Here's how the part is built. I have some questions about the finished solid (model axes, mm). A direction names the side the tool comes from. Give positions to 0.01 mm unless a question says otherwise; leave off trailing zeros. Loops run counter-clockwise (first coordinate to the right, second up) from the corner with the lowest first, then second, coordinate; pieces in that order, holes last. Notation, with made-up numbers: (67, 78.25) - (81, 78.25) arc R21 ccw to (81, 114.25) - close; hole circle Ø7 at (-9, 68.25). An arc over 180 degrees is marked (long way). Put each result on its own line as item: value. Start each with the question number.
Autodesk Inventor part; units mm, degrees
ref_plane "YZ Plane" through (0, 0, 0) normal (1, 0, 0) x (0, 1, 0)
ref_plane "XZ Plane" through (0, 0, 0) normal (0, 1, 0) x (-1, 0, 0)
ref_plane "XY Plane" through (0, 0, 0) normal (0, 0, 1) x (1, 0, 0)
sketch "スケッチ1" plane through (0, 0, 0) normal (0, 0, 1) x (1, 0, 0)
  line L0 (0, 0) -> (80, 0)
  line L1 (80, 0) -> (80, 45)
  line L2 (80, 45) -> (0, 45)
  line L3 (0, 45) -> (0, 0)
  dimension "d0" = 80
  dimension "d1" = 45
extrude "押し出し1" add sketch "スケッチ1" along normal blind 3
sketch "スケッチ2" plane through (0, 0, 3) normal (0, 0, 1) x (1, 0, 0)
  line L0 (0, 45) -> (0, 0)
  line L1 (0, 0) -> (80, 0)
  line L2 (80, 45) -> (0, 45)
  line L3 (40, 45) -> (40, 0) construction
  point P0 (7.5, 35)
  point P1 (7.5, 25)
  point P2 (30, 7.5)
  point P3 (72.5, 35)
  point P4 (72.5, 25)
  point P5 (50, 7.5)
  point P6 (40, 7.5)
  dimension "d4" = 7.5
  dimension "d5" = 35
  dimension "d6" = 10
  dimension "d7" = 7.5
  dimension "d8" = 7.5
  dimension "d9" = 30
hole "穴1" at (7.5, 35, 3) at (7.5, 25, 3) at (30, 7.5, 3) at (72.5, 35, 3) at (72.5, 25, 3) at (50, 7.5, 3) at (40, 7.5, 3) direction (0, 0, -1) diameter 3.2 end through all
sketch "スケッチ3" plane through (0, 0, 3) normal (0, 0, 1) x (1, 0, 0)
  line L0 (80, 45) -> (0, 45)
  line L1 (15, 45) -> (65, 45)
  line L2 (65, 45) -> (65, 15)
  line L3 (65, 15) -> (15, 15)
  line L4 (15, 15) -> (15, 45)
  line L5 (0, 45) -> (0, 0)
  line L6 (0, 0) -> (80, 0)
  dimension "d17" = 50
  dimension "d18" = 30
  dimension "d19" = 15
  dimension "d20" = 15
extrude "押し出し2" cut sketch "スケッチ3" against normal blind 3
fillet "フィレット1" radius 2 8 edges at (15, 45, 1.5) (65, 15, 1.5) (65, 45, 1.5) (80, 45, 1.5) (0, 45, 1.5) (0, 0, 1.5) (80, 0, 1.5) (15, 15, 1.5)
properties part number "射出_固定1" material "アルミニウム 6061"
1) Which directions (+Z, -Z, +X, -X, +Y, -Y) give clear straight access to the entire face, cutting with the end or side of a thin tool? Please do faces 4 (the flat face through (65, 30, 2)), 5 (the cylindrical face through (70.914, 25.208, 1.479)).
2) I'm going to push a flat-ended pin straight in: P1, Ø3, axis at x = 40, y = 7.5, coming from the +Z side. Where does the tip first touch, or does it pass through?
3) Suppose I cut it at B-B on y = 7.5. Please give me the cut outline in (x, z).
4) Suppose I cut it at D-D on z = 2.2. Please give me the cut outline in (x, y).
5) Suppose I cut it at A-A on y = 30. Please give me the cut outline in (x, z).
6) I need wall thicknesses on line 1 (X direction, y = 7.5, z = 2.1); line 2 (Y direction, x = 7.5, z = 1.5); line 3 (Y direction, x = 40, z = 1.3). Which ranges of each line are inside material? Lowest first, please.
7) Suppose I cut it at C-C on x = 30. Please give me the cut outline in (y, z).
8) Thinking about a two-plate mould opening in X: for faces 1 (the cylindrical face through (41.42, 6.76, 1.48)), 2 (the flat face through (39, 0, 1)), 3 (the cylindrical face through (79.43, 44.4, 1.52)), which applies, pulls with the +X half, pulls with the -X half, needs draft (parallel to the pull), parting line crosses it, or undercut?
Ans:
1. face 4: +Z, -Z, +Y
1. face 5: +Z, -Z
2. P1: passes through
3. outline: (0, 0) - (28.4, 0) - (28.4, 3) - (0, 3) - close; (31.6, 0) - (38.4, 0) - (38.4, 3) - (31.6, 3) - close; (41.6, 0) - (48.4, 0) - (48.4, 3) - (41.6, 3) - close; (51.6, 0) - (80, 0) - (80, 3) - (51.6, 3) - close
4. outline: (0, 2) arc R2 ccw to (2, 0) - (78, 0) arc R2 ccw to (80, 2) - (80, 43) arc R2 ccw to (78, 45) - (67, 45) arc R2 ccw to (65, 43) - (65, 17) arc R2 cw to (63, 15) - (17, 15) arc R2 cw to (15, 17) - (15, 43) arc R2 ccw to (13, 45) - (2, 45) arc R2 ccw to (0, 43) - close; hole circle Ø3.2 at (7.5, 25); hole circle Ø3.2 at (7.5, 35); hole circle Ø3.2 at (30, 7.5); hole circle Ø3.2 at (40, 7.5); hole circle Ø3.2 at (50, 7.5); hole circle Ø3.2 at (72.5, 25); hole circle Ø3.2 at (72.5, 35)
5. outline: (0, 0) - (15, 0) - (15, 3) - (0, 3) - close; (65, 0) - (80, 0) - (80, 3) - (65, 3) - close
6. line 1: x = 0 to 28.4, 31.6 to 38.4, 41.6 to 48.4, 51.6 to 80
6. line 2: y = 0 to 23.4, 26.6 to 33.4, 36.6 to 45
6. line 3: y = 0 to 5.9, 9.1 to 15
7. outline: (0, 0) - (5.9, 0) - (5.9, 3) - (0, 3) - close; (9.1, 0) - (15, 0) - (15, 3) - (9.1, 3) - close
8. face 1: undercut
8. face 2: needs draft
8. face 3: pulls with the +X half
